Work out the finished part from the listing and answer in its coordinate system (mm). Face numbers are marked on the shaded views. A direction names the side the tool comes from. Round coordinates to 2 decimals unless told otherwise and drop trailing zeros. Order: outer loops, then holes, each group sorted by start corner. A loop starts at its lowest first (then second) coordinate and runs counter-clockwise, first axis right, second up. Notation, with made-up numbers: M 38.25,73 L 71.25,73 A24 cw 71.25,96 Z; hole C -11.75,16.25 d6. An arc over 180 degrees is marked long. Return JSON: item names as keys, results as strings.
Autodesk Inventor part; units mm, degrees
ref_plane "作業平面1" through (-27.3255, 41.0319, 38.0074) normal (1, 0, 0) x (0, 1, 0)
ref_plane "作業平面2" through (73.5745, 41.0319, 11.4574) normal (0, -1, 0) x (1, 0, 0)
ref_plane "YZ Plane" through (0, 0, 0) normal (1, 0, 0) x (0, 1, 0)
ref_plane "作業平面1" through (-27.3255, 41.0319, 38.0074) normal (1, 0, 0) x (0, 1, 0)
sketch "スケッチ2" plane through (-27.3255, 41.0319, 38.0074) normal (1, 0, 0) x (0, 1, 0)
  arc A0 (-51.6, -13.3) -> (-38.35, -26.55) centre (-38.35, -13.3) ccw
  line L0 (-51.6, 0) -> (-51.6, -13.3)
  arc A1 (-51.6, 0) -> (-38.35, -13.25) centre (-38.35, 0) ccw
  line L1 (38.35, -13.25) -> (-38.35, -13.25)
  arc A2 (38.35, -13.25) -> (51.6, 0) centre (38.35, 0) ccw
  line L2 (51.6, -13.3) -> (51.6, 0)
  arc A3 (38.35, -26.55) -> (51.6, -13.3) centre (38.35, -13.3) ccw
  line L3 (-38.35, -26.55) -> (38.35, -26.55)
  point P0 (-41.0319, -38.0074)
extrude "押し出し1" add sketch "スケッチ2" along normal blind 100.9
sketch "スケッチ3" plane through (-27.3255, 2.6819, 11.4574) normal (0, 0, -1) x (-1, 0, 0)
  line L0 (0, 76.7) -> (-100.9, 76.7)
  line L1 (-100.9, 0) -> (-100.9, 76.7)
  line L2 (0, 0) -> (-100.9, 0)
  line L3 (0, 76.7) -> (0, 0)
  point P0 (-27.3255, -2.6819)
  point P1 (-90.9, 66.7)
  point P2 (-90.9, 10)
  point P3 (-15, 10)
  point P4 (-15, 66.7)
  dimension "d2" = 10
  dimension "d3" = 10
  dimension "d4" = 10
  dimension "d5" = 10
  dimension "d6" = 10
  dimension "d7" = 15
  dimension "d8" = 15
  dimension "d9" = 10
hole "穴2" at (63.5745, 69.3819, 11.4574) at (63.5745, 12.6819, 11.4574) at (-12.3255, 12.6819, 11.4574) at (-12.3255, 69.3819, 11.4574) direction (0, 0, 1) diameter 4.2 depth 10.979 tip angle 118
sketch "スケッチ4" plane through (-27.3255, 2.6819, 11.4574) normal (0, 0, -1) x (-1, 0, 0)
  circle A0 centre (-34.275, 38.35) radius 4.175
  circle A1 centre (-34.275, 38.35) radius 3.35
  point P0 (-27.3255, -2.6819)
  dimension "d24" = 6.7
  dimension "d44" = 8.35
hole "穴3" [suppressed]
sketch "スケッチ6" plane through (73.5745, 41.0319, 38.0074) normal (1, 0, 0) x (0, 0, -1)
  line L0 (0, -51.6) -> (13.3, -51.6)
  line L1 (13.3, 51.6) -> (0, 51.6)
  line L2 (26.55, -38.35) -> (26.55, 38.35)
  arc A0 (13.3, 51.6) -> (17.3, 55.6) centre (13.3, 55.6) ccw
  line L3 (17.3, 55.6) -> (17.3, 65.9409)
  line L4 (17.3, 65.9409) -> (26.55, 65.9409)
  line L5 (26.55, 65.9409) -> (26.55, 38.35)
  line L6 (26.55, 0) -> (-17.064, 0) construction
  arc A1 (17.3, -55.6) -> (13.3, -51.6) centre (13.3, -55.6) ccw
  line L7 (17.3, -55.6) -> (17.3, -65.9409)
  line L8 (17.3, -65.9409) -> (26.55, -65.9409)
  line L9 (26.55, -65.9409) -> (26.55, -38.35)
  arc A2 (13.3, -51.6) -> (26.55, -38.35) centre (13.3, -38.35) ccw
  arc A3 (26.55, 38.35) -> (13.3, 51.6) centre (13.3, 38.35) ccw
  point P0 (38.0074, -41.0319)
  dimension "d32" = 90
  dimension "d34" = 4
  dimension "d35" = 38.35
extrude "押し出し2" add sketch "スケッチ6" against normal blind 124.8
ref_plane "作業平面2" through (73.5745, 41.0319, 11.4574) normal (0, -1, 0) x (1, 0, 0)
sketch "スケッチ8" plane through (-27.3255, 2.6819, 11.4574) normal (0, 0, -1) x (-1, 0, 0)
  circle A0 centre (-34.275, 38.35) radius 4.175
  circle A1 centre (-34.275, 38.35) radius 4.175
  circle A2 centre (-34.275, 38.35) radius 4.175
  circle A3 centre (-34.275, 38.35) radius 3.375
  circle A4 centre (-34.275, 38.35) radius 6.7437
  circle A5 centre (-34.275, 38.35) radius 7
  point P0 (-27.3255, -2.6819)
  point P1 (-34.275, 38.35)
  dimension "d65" = 14
sketch "スケッチ9" plane through (-27.3255, 2.6819, 11.4574) normal (0, 0, -1) x (-1, 0, 0)
  circle A0 centre (-15, 66.7) radius 2.1
  circle A1 centre (-15, 10) radius 2.1
  circle A2 centre (-90.9, 10) radius 2.1
  circle A3 centre (-90.9, 66.7) radius 2.1
  line L0 (48.86, 38.35) -> (-125.86, 38.35)
  line L1 (-100.9, 104.2909) -> (23.9, 104.2909)
  line L2 (0, 89.95) -> (-100.9, 89.95)
  point P0 (-27.3255, -2.6819)
  point P1 (-52.9, 97.1909)
  point P2 (-52.9, -20.4909)
  dimension "d54" = 38
  dimension "d55" = 7.1
hole "穴5" at (25.5745, 99.8728, 11.4574) at (25.5745, -17.809, 11.4574) direction (0, 0, 1) diameter 4.2 depth 6 tip angle 118
extrude "押し出し4" cut sketch "スケッチ8" against normal blind 8.17 contours A0 | A3 | A4 | A5
sketch "スケッチ11" plane through (6.9495, 41.0319, 19.6274) normal (0, 0, -1) x (-1, 0, 0)
  circle A0 centre (0, 0) radius 7
  point P0 (6.9495, -41.0319)
hole "穴6" at (6.9495, 41.0319, 19.6274) direction (0, 0, 1) diameter 5 depth 6 tip angle 118 countersink diameter 14 countersink angle 90
properties part number "AzureKinectCradle"
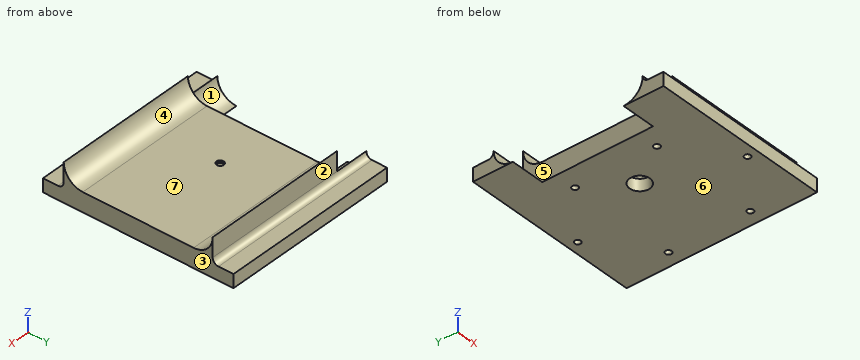
Item 1: Find section D-D (y = 84). Determine the outline of the cut face in (x, z).
Output:
{"outline": "M -51.23,11.46 L 73.57,11.46 L 73.57,25.59 L -27.33,25.59 L -27.33,12.29 L -51.23,12.29 Z"}
Item 2: Each of these flat-tipped pins is pushed along its axis until it touches: pin 1 (8.5 mm diameter, centred on x = -7.5, y = 102.5, fed in from +Z); pin 2 (2.5 mm diameter, centred on x = -12.33, y = 12.68, fed in from +Z); pin 3 (2.5 mm diameter, centred on x = 63.57, y = 12.68, fed in from -Z); pin 4 (5.5 mm diameter, centred on x = 25.57, y = 99.87, fed in from -Z). Where does it stop, or does it pass through?
Output:
{"pin 1": "stops at z = 20.71", "pin 2": "stops at z = 24.76", "pin 3": "stops at z = 22.94", "pin 4": "stops at z = 11.46"}
Item 3: Consider line 1 along X through (y, z) = (68, 22.5); line 2 along Z through (x, y) = (-17, 20.5); line 3 along Y through (x, z) = (-38.5, 23.25). Determine where each line is inside the solid, lowest interval first. Write a range as [from, to].
Output:
{"line 1": "x = [-27.33, -13.76], [-10.89, 62.14], [65.01, 73.57]", "line 2": "z = [11.46, 24.76]", "line 3": "y = [-10.84, -10.49], [92.55, 92.91]"}
Item 4: Find section A-A (x = -37). Determine the outline of the cut face in (y, z), plus the area to 3 significant figures.
Output:
{"outline": "M -24.91,11.46 L 2.68,11.46 A13.25 cw -10.57,24.71 A4 cw -14.57,20.71 L -24.91,20.71 Z; M 79.38,11.46 L 106.97,11.46 L 106.97,20.71 L 96.63,20.71 A4 cw 92.63,24.71 A13.25 cw Z", "area": "348 mm^2"}
Item 5: Which of the six approach directions +Z, -Z, +X, -X, +Y, -Y give full straight-line access (tool end or side, diameter ignored) to the marked faces 5, 6 and 7?
Output:
{"face 5": "+Z, -X", "face 6": "-Z, +X, -X, +Y, -Y", "face 7": "+Z, +X, -X"}
Item 6: Find section C-C (x = 29.5). Determine the outline of the cut face in (y, z).
Output:
{"outline": "M -24.91,11.46 L 106.97,11.46 L 106.97,20.71 L 96.63,20.71 A4 cw 92.63,24.71 L 92.63,38.01 A13.25 cw 79.38,24.76 L 2.68,24.76 A13.25 cw -10.57,38.01 L -10.57,24.71 A4 cw -14.57,20.71 L -24.91,20.71 Z"}
Item 7: Find section B-B (z = 32.5). Determine the outline of the cut face in (x, y), plus the area to 3 significant figures.
Output:
{"outline": "M -27.33,-10.57 L 73.57,-10.57 L 73.57,-9.37 L -27.33,-9.37 Z; M -27.33,91.43 L 73.57,91.43 L 73.57,92.63 L -27.33,92.63 Z", "area": "242 mm^2"}
Item 8: The mould has two halves that part along Y. Classify the marked faces 1, 2, 3 and 4: pulls with the +Y half, pulls with the -Y half, needs draft (parallel to the pull), parting line crosses it, or undercut.
Output:
{"face 1": "undercut", "face 2": "pulls with the +Y half", "face 3": "needs draft", "face 4": "undercut"}
